```python
from build123d import *

# Parameters (mm, degrees)
SKETCH1_W           = 25.4
SKETCH1_H           = 25.4
SKETCH1_R           = 3.2639
BOSS_EXTRUDE1_DEPTH = 3.175
SKETCH2_W           = 25.4
SKETCH2_H           = 3.175
BOSS_EXTRUDE2_DEPTH = 22.225
SKETCH3_R           = 3.2639
CUT_EXTRUDE1_DEPTH  = 3.175
FILLET1_R           = 3.175


with BuildPart() as part:
    # Sketch1 → Boss-Extrude1 (new body)
    with BuildSketch(Plane(origin=(0, 0, 0), x_dir=(1, 0, 0), z_dir=(0, 1, 0))):
        with Locations((12.7, 12.7)):
            Rectangle(SKETCH1_W, SKETCH1_H)
        with Locations((12.7, 12.7)):
            Circle(SKETCH1_R, mode=Mode.SUBTRACT)
    extrude(amount=BOSS_EXTRUDE1_DEPTH)

    # Sketch2 → Boss-Extrude2 (add)
    with BuildSketch(Plane(origin=(0, 3.175, 0), x_dir=(1, 0, 0), z_dir=(0, 1, 0))):
        with Locations((12.7, 1.5875)):
            Rectangle(SKETCH2_W, SKETCH2_H)
    extrude(amount=BOSS_EXTRUDE2_DEPTH)

    # Sketch3 → Cut-Extrude1 (cut)
    with BuildSketch(Plane.XY):
        with Locations((12.7, 12.7)):
            Circle(SKETCH3_R)
    extrude(amount=-CUT_EXTRUDE1_DEPTH, mode=Mode.SUBTRACT)

    # Fillet1
    fillet1_edges = [part.edges().sort_by_distance(p)[0] for p in [
        (0, 25.4, -1.5875),
        (25.4, 25.4, -1.5875),
        (0, 1.5875, -25.4),
        (25.4, 1.5875, -25.4),
    ]]
    fillet(fillet1_edges, radius=FILLET1_R)


solid = part.part
```
The listing builds one solid part. Answer for the finished solid, in the listing's coordinates (mm). A direction names the side the tool comes from. Coordinates: 2 decimals unless noted, no trailing zeros. Loops run counter-clockwise (first coordinate to the right, second up) from the corner with the lowest first, then second, coordinate; pieces in that order, holes last. Notation, with made-up numbers: M 69,12.5 L 76,12.5 A22 cw 76,19.5 Z; hole C 4,-30 d8. An arc over 180 degrees is marked long. Answer as a JSON object with one key per item and string values. Group by question number.
Item 1: Section D-D (z = -12.7) is taken. Write down the section's boundary in (x, y) (3 decimals), and give its area (3 significant figures).
Item 2: Section A-A (y = 12.7) is taken. Write down the section's boundary in (x, z) (3 decimals), and give its area (3 significant figures).
Item 3: Section C-C (z = -1.5) is taken. Write down the section's boundary in (x, y) (3 decimals).
Item 4: Consider L1, parallel to Y at x = 12.5, z = -2.75; L2, parallel to Z at x = 12.7, y = 1.6; L3, parallel to Z at x = 1.5, y = 22.75 (3 decimals). Determine where each line is inside the solid, lowest interval first.
Item 5: Each of these flat-tipped pins is pushed along its axis until it touches: P1, Ø6, axis at x = 6.5, y = 12.5, coming from the -Z side (3 decimals); P2, Ø6, axis at x = 12.7, y = 12.7, coming from the +Z side; P3, Ø6.5, axis at x = 11.5, z = -13.5, coming from the +Y side (3 decimals). Where does it stop, or does it pass through?
Item 6: Section B-B (x = 12.7) is taken. Write down the section's boundary in (y, z) (3 decimals), and give its area (3 significant figures).
Item 7: Which of the six approach directions +Z, -Z, +X, -X, +Y, -Y give full straight-line access (tool end or side, diameter ignored) to faces 5 (the face through (0.91, 1.61, -24.45)), 6 (the face through (13, 3.175, -17))?
Item 8: Determine the mould class of faces 1 (the face through (10.11, 1.565, -10.714)), 2 (the face through (0, 3, -6)), 3 (the face through (10.11, 10.714, -1.565)), 4 (the face through (15, 0, -10)) for opening direction X: +X half, -X half, draft (parallel to the pull), parting line (faces both ways), or undercut.
Solved:
{
 "1": {"outline": "M 0,0 L 9.436,0 L 9.436,3.175 L 0,3.175 Z; M 15.964,0 L 25.4,0 L 25.4,3.175 L 15.964,3.175 Z", "area": "59.9 mm2"},
 "2": {"outline": "M 0,-3.175 L 9.436,-3.175 L 9.436,0 L 0,0 Z; M 15.964,-3.175 L 25.4,-3.175 L 25.4,0 L 15.964,0 Z", "area": "59.9 mm2"},
 "3": {"outline": "M 0,0 L 25.4,0 L 25.4,22.225 A3.175 ccw 22.225,25.4 L 3.175,25.4 A3.175 ccw 0,22.225 Z; hole C 12.7,12.7 d6.528"},
 "4": {"L1": "y = 0 to 9.44, 15.96 to 25.4", "L2": "z = -25.4 to -15.96, -9.44 to 0", "L3": "z = -3.175 to 0"},
 "5": {"P1": "stops at z = -3.175", "P2": "passes through", "P3": "stops at y = 3.175"},
 "6": {"outline": "M 0,-25.4 L 3.175,-25.4 L 3.175,-15.964 L 0,-15.964 Z; M 0,-9.436 L 3.175,-9.436 L 3.175,-3.175 L 9.436,-3.175 L 9.436,0 L 0,0 Z; M 15.964,-3.175 L 25.4,-3.175 L 25.4,0 L 15.964,0 Z", "area": "110 mm2"},
 "7": {"face 5": "-Z, -X, +Y, -Y", "face 6": "-Z, +X, -X, +Y"},
 "8": {"face 1": "undercut", "face 2": "-X half", "face 3": "undercut", "face 4": "draft"}
}
